For this review, take the finished solid that the model builds, in its own axes (mm). A direction names the side the tool comes from. Coordinates: 2 decimals unless noted, no trailing zeros. Write each loop counter-clockwise with the first axis right and the second up, starting at its lowest first coordinate (ties: lowest second). Pieces come first, ordered by that corner, then holes.
```python
from build123d import *

# Parameters (mm, degrees)
BOSS_EXTRUDE1_DEPTH = 15
SKETCH2_R           = 5
BOSS_EXTRUDE2_DEPTH = 61


with BuildPart() as part:
    # Sketch1 → Boss-Extrude1 (new body)
    with BuildSketch(Plane.YZ):
        Polygon((0, 0), (0, 95), (60, 95), (60, 120), (-30, 120), (-30, -25), (60, -25), (60, 0), align=None)
    extrude(amount=BOSS_EXTRUDE1_DEPTH)

    # Sketch2 → Boss-Extrude2 (add)
    with BuildSketch(Plane(origin=(0, 0, 95), x_dir=(1, 0, 0), z_dir=(0, 0, -1))):
        with Locations(Location((7.5, -52.5, 0), (0, 0, 90))):
            Circle(SKETCH2_R)
    extrude(amount=BOSS_EXTRUDE2_DEPTH)


solid = part.part
```
1) Consider section B-B (z = 87.5). Give the boundary of the cut face in (x, y).
2) Consider section D-D (y = 52.5). Give the boundary of the cut face in (x, z).
3) Consider section C-C (x = 7.5). Give the boundary of the cut face in (y, z).
4) The part is to be moulded in two halves that separate along Y. For faces 1 (the face through (7, 0, 47)), 2 (the face through (7, 30, 0)), 3 (the face through (7, 60, -13)), say which applies: pulls with the +Y half, pulls with the -Y half, needs draft (parallel to the pull), parting line crosses it, or undercut.
5) Clearance check with flat-ended pins moving along their axes: P1, Ø4, axis at x = 5.5, z = 58, coming from the +Y side; P2, Ø8, axis at x = 9.5, z = 29, coming from the +Y side. State where each tip first meets the part, or that it passes through.
6) Consider section A-A (y = 31). Give the boundary of the cut face in (x, z), then the cut area to 3 significant figures.
7) For L1, parallel to Y at x = 7, z = 45; L2, parallel to Z at x = 5.25, y = 34.5; L3, parallel to Z at x = 7.75, y = 54.5, list the stretches that pass through material, from the lowest coordinate up.
8) Tool access review of faces 4 (the face through (7, 53, 34)), 5 (the face through (0, -6, 49)), 6 (the face through (7.28, 57.495, 64.927)): name each direction out of +Z, -Z, +X, -X, +Y, -Y from which nothing blocks a thin tool from reaching the whole face with its end or side.
Results:
1. outline: (0, -30) - (15, -30) - (15, 0) - (0, 0) - close; circle Ø10 at (7.5, 52.5)
2. outline: (0, -25) - (15, -25) - (15, 0) - (0, 0) - close; (0, 95) - (2.5, 95) - (2.5, 34) - (12.5, 34) - (12.5, 95) - (15, 95) - (15, 120) - (0, 120) - close
3. outline: (-30, -25) - (60, -25) - (60, 0) - (0, 0) - (0, 95) - (47.5, 95) - (47.5, 34) - (57.5, 34) - (57.5, 95) - (60, 95) - (60, 120) - (-30, 120) - close
4. face 1: undercut
4. face 2: needs draft
4. face 3: pulls with the +Y half
5. P1: stops at y = 57.5
5. P2: stops at y = 0
6. outline: (0, -25) - (15, -25) - (15, 0) - (0, 0) - close; (0, 95) - (15, 95) - (15, 120) - (0, 120) - close
6. area: 750 mm2
7. L1: y = -30 to 0, 47.53 to 57.47
7. L2: z = -25 to 0, 95 to 120
7. L3: z = -25 to 0, 34 to 120
8. face 4: +X, -X, +Y
8. face 5: +Z, -Z, -X, +Y, -Y
8. face 6: none
